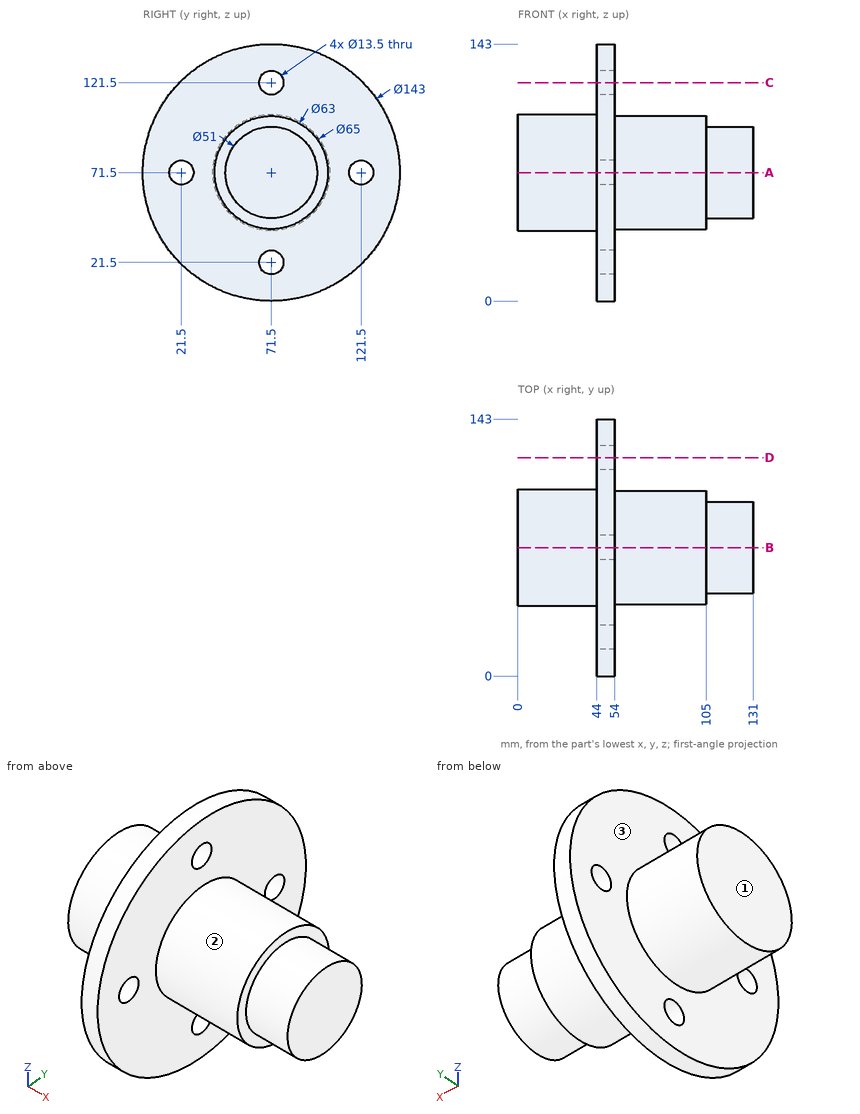
Geometry check sheet. Reference: drawing and pictorial views, mm from the part's lowest x, y, z. A direction names the side the tool comes from. Give positions to 0.01 mm unless a question says otherwise; leave off trailing zeros. Order: outer loops, then holes, each group sorted by start corner. A loop starts at its lowest first (then second) coordinate and runs counter-clockwise, first axis right, second up. Notation, with made-up numbers: M -9,20 L 9,20 A16 ccw 9,35 Z; hole C 20.5,4 d9. An arc over 180 degrees is marked long. Answer in a Markdown table with one row per item. Add a question column.
Q1. Access from +Z, -Z, +X, -X, +Y, -Y to the whole of each face (thin tool, end or side, straight path). Record for the marked faces 1, 2 and 3.
Q2. Gauge pin test, flat ends, axial feed: pin 1 Ø8 at (y, z) = (71.5, 21.5) entering from -X; pin 2 Ø5 at (x, z) = (106.5, 67) entering from +Y; pin 3 Ø12 at (y, z) = (116.5, 99.5) entering from -X; pin 4 Ø3 at (x, z) = (26, 59) entering from +Y. Record the tip position at first contact, or that the pin passes through.
Q3. Sectioned sample at A-A, the plane z = 71.5. Record the boundary of the cut face in (x, y).
Q4. Thickness scan on L1, parallel to Y at x = 48, z = 71.5; L2, parallel to X at y = 26, z = 81; L3, parallel to X at y = 69, z = 103. Record the ranges inside material, lowest first.
Q5. Sectioned sample at C-C, the plane z = 121.5. Record the boundary of the cut face in (x, y), and give its area (3 significant figures).
Verdict:
| question | item | result |
|---|---|---|
| 1 | face 1 | +Z, -Z, -X, +Y, -Y |
| 1 | face 2 | +X |
| 1 | face 3 | -X |
| 2 | pin 1 | through |
| 2 | pin 2 | y = 102.9 |
| 2 | pin 3 | x = 44 |
| 2 | pin 4 | y = 102.08 |
| 3 | outline | M 0,39 L 44,39 L 44,28.25 L 54,28.25 L 54,40 L 105,40 L 105,46 L 131,46 L 131,97 L 105,97 L 105,103 L 54,103 L 54,114.75 L 44,114.75 L 44,104 L 0,104 Z; M 44,0 L 54,0 L 54,14.75 L 44,14.75 Z; M 44,128.25 L 54,128.25 L 54,143 L 44,143 Z |
| 4 | L1 | 0 to 14.75, 28.25 to 114.75, 128.25 to 143 |
| 4 | L2 | 44 to 54 |
| 4 | L3 | 0 to 54 |
| 5 | outline | M 44,20.39 L 54,20.39 L 54,64.75 L 44,64.75 Z; M 44,78.25 L 54,78.25 L 54,122.61 L 44,122.61 Z |
| 5 | area | 887 mm² |
